```python
from build123d import *

# Parameters (mm, degrees)
SKETCH_W            = 80
SKETCH_H            = 120
PAD_DEPTH           = 3
SKETCH001_W         = 70
SKETCH001_H         = 110
POCKET_DEPTH        = 2
SKETCH002_W         = 62
SKETCH002_H         = 98.5
POCKET001_DEPTH     = 5
FILLET_R            = 2.54
CHAMFER_SIZE        = 1.99
SKETCH003_W         = 126
SKETCH003_H         = 60
PAD001_DEPTH        = 3
SKETCH004_W         = 80
SKETCH004_H         = 60
PAD002_DEPTH        = 3
CHAMFER001_SIZE     = 9.5
SKETCH005_R         = 1.8
POCKET002_DEPTH     = 8
FILLET001_R         = 2.99
SKETCH006_W         = 8
SKETCH006_H         = 10
PAD003_DEPTH        = 10
SKETCH007_W         = 8
SKETCH007_H         = 10
PAD004_DEPTH        = 20
SKETCH008_R         = 1.4
POCKET003_DEPTH     = 7
SKETCH009_R         = 1.4
POCKET004_DEPTH     = 7
CHAMFER002_SIZE     = 9.99
CHAMFER003_SIZE     = 9.99
CHAMFER004_SIZE     = 1.49
CHAMFER005_SIZE     = 6
CHAMFER005_FACE36_R = 1.4
POCKET005_DEPTH     = 2
POCKET005_FACE45_R  = 1.4
POCKET006_DEPTH     = 2
POCKET006_FACE2_R   = 1.4
POCKET007_DEPTH     = 2
POCKET007_FACE55_R  = 1.4
POCKET008_DEPTH     = 2
FILLET002_R         = 3.99


with BuildPart() as part:
    # Sketch → Pad (new body)
    with BuildSketch(Plane.XY):
        Rectangle(SKETCH_W, SKETCH_H)
    extrude(amount=PAD_DEPTH)

    # Sketch001 (on Face6 of Pad) → Pocket (cut)
    with BuildSketch(Plane.XY.offset(3)):
        Rectangle(SKETCH001_W, SKETCH001_H)
    extrude(amount=-POCKET_DEPTH, mode=Mode.SUBTRACT)

    # Sketch002 (on Face11 of Pocket) → Pocket001 (cut)
    with BuildSketch(Plane.XY.offset(1)):
        Rectangle(SKETCH002_W, SKETCH002_H)
    extrude(amount=-POCKET001_DEPTH, mode=Mode.SUBTRACT)

    # Fillet
    fillet_edges = [part.edges().sort_by_distance(p)[0] for p in [
        (-31, 49.25, 0.5),
        (31, 49.25, 0.5),
        (31, -49.25, 0.5),
        (-31, -49.25, 0.5),
    ]]
    fillet(fillet_edges, radius=FILLET_R)

    # Chamfer
    chamfer_edges = [part.edges().sort_by_distance(p)[0] for p in [
        (0, 55, 1),
        (35, 0, 1),
        (0, -55, 1),
        (-35, 0, 1),
    ]]
    chamfer(chamfer_edges, length=CHAMFER_SIZE)

    # Sketch003 (on Face22 of Chamfer) → Pad001 (join)
    with BuildSketch(Plane.YZ.offset(40)):
        with Locations((0, 30)):
            Rectangle(SKETCH003_W, SKETCH003_H)
    pad001 = extrude(amount=PAD001_DEPTH)

    # Mirrored: Pad001 across YZ
    add(pad001.mirror(Plane.YZ))

    # Sketch004 (on Face9 of Mirrored) → Pad002 (join)
    with BuildSketch(Plane(origin=(0, 60, 0), x_dir=(-1, 0, 0), z_dir=(0, 1, 0))):
        with Locations((0, 30)):
            Rectangle(SKETCH004_W, SKETCH004_H)
    pad002 = extrude(amount=PAD002_DEPTH)

    # Mirrored001: Pad002 across XZ
    add(pad002.mirror(Plane.XZ))

    # Chamfer001
    chamfer001_edges = [part.edges().sort_by_distance(p)[0] for p in [
        (-40, -60, 31.5),
        (-40, 60, 31.5),
        (40, 60, 31.5),
        (40, -60, 31.5),
    ]]
    chamfer(chamfer001_edges, length=CHAMFER001_SIZE)

    # Sketch005 (on Face4 of Chamfer001) → Pocket002 (cut)
    with BuildSketch(Plane.XY.offset(60)):
        with Locations((-38.403806, -58.403806)):
            Circle(SKETCH005_R)
        with Locations((38.403806, -58.403806)):
            Circle(SKETCH005_R)
    pocket002 = extrude(amount=-POCKET002_DEPTH, mode=Mode.SUBTRACT)

    # Mirrored002: Pocket002 across XZ
    add(pocket002.mirror(Plane.XZ), mode=Mode.SUBTRACT)

    # Fillet001
    fillet001_edges = [part.edges().sort_by_distance(p)[0] for p in [
        (-43, 63, 30),
        (-43, -63, 30),
        (43, -63, 30),
        (43, 63, 30),
    ]]
    fillet(fillet001_edges, radius=FILLET001_R)

    # Sketch006 (on Face21 of Fillet001) → Pad003 (join)
    with BuildSketch(Plane(origin=(0, -60, 0), x_dir=(-1, 0, 0), z_dir=(0, 1, 0))):
        with Locations((-25, 25)):
            Rectangle(SKETCH006_W, SKETCH006_H)
        with Locations((25, 25)):
            Rectangle(SKETCH006_W, SKETCH006_H)
    extrude(amount=PAD003_DEPTH)

    # Sketch007 (on Face10 of Pad003) → Pad004 (join)
    with BuildSketch(Plane.YZ.offset(-40)):
        with Locations((-4, 25)):
            Rectangle(SKETCH007_W, SKETCH007_H)
    pad004 = extrude(amount=PAD004_DEPTH)

    # Sketch008 (on Face41 of Pad004) → Pocket003 (cut)
    with BuildSketch(Plane.XY.offset(30)):
        with Locations((-25, -54)):
            Circle(SKETCH008_R)
    pocket003 = extrude(amount=-POCKET003_DEPTH, mode=Mode.SUBTRACT)

    # Mirrored003: Pocket003 across Sketch008 V_Axis
    add(pocket003.mirror(Plane(origin=(0, 0, 30), x_dir=(0, 0, 1), z_dir=(1, 0, 0))), mode=Mode.SUBTRACT)

    # Sketch009 (on Face26 of Mirrored003) → Pocket004 (cut)
    with BuildSketch(Plane.XY.offset(30)):
        with Locations((-25, -4)):
            Circle(SKETCH009_R)
    pocket004 = extrude(amount=-POCKET004_DEPTH, mode=Mode.SUBTRACT)

    # Mirrored004: Pad004 across YZ
    add(pad004.mirror(Plane.YZ))

    # Mirrored005: Pocket004 across Sketch009 V_Axis
    add(pocket004.mirror(Plane(origin=(0, 0, 30), x_dir=(0, 0, 1), z_dir=(1, 0, 0))), mode=Mode.SUBTRACT)

    # Chamfer002
    chamfer002_edges = [part.edges().sort_by_distance(p)[0] for p in [
        (25, -60, 20),
        (-25, -60, 20),
    ]]
    chamfer(chamfer002_edges, length=CHAMFER002_SIZE)

    # Chamfer003
    chamfer003_edges = [part.edges().sort_by_distance(p)[0] for p in [
        (40, -4, 20),
        (-40, -4, 20),
    ]]
    chamfer(chamfer003_edges, length=CHAMFER003_SIZE)

    # Chamfer004
    chamfer004_edges = [part.edges().sort_by_distance(p)[0] for p in [
        (29, -60, 15.005),
        (29, -60, 25),
        (-29, -60, 15.005),
        (-21, -60, 15.005),
        (21, -60, 15.005),
    ]]
    chamfer(chamfer004_edges, length=CHAMFER004_SIZE)

    # Chamfer005
    chamfer005_edges = [part.edges().sort_by_distance(p)[0] for p in [
        (-40, 0, 15.005),
        (-40, -8, 15.005),
        (40, -8, 15.005),
        (40, 0, 15.005),
    ]]
    chamfer(chamfer005_edges, length=CHAMFER005_SIZE)

    # Chamfer005 Face36 → Pocket005 (cut)
    with BuildSketch(Plane(origin=(31.679222, -4, 30), x_dir=(0, 1, 0), z_dir=(0, 0, 1))):
        Polygon((-4, 11.679222), (-4, -2.320778), (-10, -8.320778), (-4, -8.320778), (4, -8.320778), (10, -8.320778), (4, -2.320778), (4, 11.679222), align=None)
        with Locations((0, 6.679222)):
            Circle(CHAMFER005_FACE36_R, mode=Mode.SUBTRACT)
    extrude(amount=-POCKET005_DEPTH, mode=Mode.SUBTRACT)

    # Pocket005 Face45 → Pocket006 (cut)
    with BuildSketch(Plane(origin=(25, -55.212396, 30), x_dir=(0, 1, 0), z_dir=(0, 0, 1))):
        Polygon((-3.297604, -4), (5.212396, -4), (5.212396, 4), (-3.297604, 4), (-4.787604, 5.49), (-4.787604, 4), (-4.787604, -4), (-4.787604, -5.49), align=None)
        with Locations((1.212396, 0)):
            Circle(POCKET005_FACE45_R, mode=Mode.SUBTRACT)
    extrude(amount=-POCKET006_DEPTH, mode=Mode.SUBTRACT)

    # Pocket006 Face2 → Pocket007 (cut)
    with BuildSketch(Plane(origin=(-31.679222, -4, 30), x_dir=(0, 1, 0), z_dir=(0, 0, 1))):
        Polygon((-4, 2.320778), (-4, -11.679222), (4, -11.679222), (4, 2.320778), (10, 8.320778), (4, 8.320778), (-4, 8.320778), (-10, 8.320778), align=None)
        with Locations((0, -6.679222)):
            Circle(POCKET006_FACE2_R, mode=Mode.SUBTRACT)
    extrude(amount=-POCKET007_DEPTH, mode=Mode.SUBTRACT)

    # Pocket007 Face55 → Pocket008 (cut)
    with BuildSketch(Plane(origin=(-25, -55.212396, 30), x_dir=(0, 1, 0), z_dir=(0, 0, 1))):
        Polygon((-3.297604, -4), (5.212396, -4), (5.212396, 4), (-3.297604, 4), (-4.787604, 5.49), (-4.787604, 4), (-4.787604, -4), (-4.787604, -5.49), align=None)
        with Locations((1.212396, 0)):
            Circle(POCKET007_FACE55_R, mode=Mode.SUBTRACT)
    extrude(amount=-POCKET008_DEPTH, mode=Mode.SUBTRACT)

    # Fillet002
    fillet002_edges = [part.edges().sort_by_distance(p)[0] for p in [
        (20, 0, 24),
        (20, -8, 24),
        (-20, -8, 24),
        (-20, 0, 24),
        (-29, -50, 24),
        (-21, -50, 24),
        (21, -50, 24),
        (29, -50, 24),
    ]]
    fillet(fillet002_edges, radius=FILLET002_R)


solid = part.part
```
Geometry check sheet. Reference: the model listing, model coordinates, mm. A direction names the side the tool comes from. Give positions to 0.01 mm unless a question says otherwise; leave off trailing zeros. Loops run counter-clockwise (first coordinate to the right, second up) from the corner with the lowest first, then second, coordinate; pieces in that order, holes last. Notation, with made-up numbers: M -2.75,77.25 L 3.25,77.25 A25 ccw 3.25,107.25 Z; hole C -15.75,74 d8. An arc over 180 degrees is marked long. Write item = value, one per line. Start each with the question number.
1. Tool access check on faces 1 (the face through (-25, -54, 23)), 2 (the face through (-43, -1, 30)), 3 (the face through (25.08, -54.94, 15.07)), 4 (the face through (-21.14, -6.8, 24.06)). Record the directions out of +Z, -Z, +X, -X, +Y, -Y that give a thin tool (end or side, any length) a straight path to the whole face; none if there is none.
2. Draft check along X on faces 5 (the face through (37, 3, 21)), 6 (the face through (-42.15, 62.1, 30.42)), 7 (the face through (39, 1, 0)). Enter one of: +X half, -X half, draft (parallel to the pull), parting line (faces both ways), or undercut.
3. Section check C-C, the plane z = 8. Enter the section's corners in (x, y), plus the area to 3 significant figures.
4. Go/stop test with flat-tipped pins: P1, Ø2, axis at x = 25, y = -54.5, coming from the +Z side; P2, Ø0.8, axis at x = -24.5, y = -3.5, coming from the +Z side. Record where each tip stops, or that it passes through.
5. Section check D-D, the plane z = 55.5. Enter the section's corners in (x, y), plus the area to 3 significant figures.
6. Thickness scan on probe 1 along Y at (x, z) = (25, 24.7); probe 2 along X at (y, z) = (-4, 26.6); probe 3 along X at (y, z) = (-5, 57). Record the ranges inside material, lowest first.
Values follow:
q1.face_1 = +Z
q1.face_2 = +Z, -Z, -X, +Y, -Y
q1.face_3 = none
q1.face_4 = +Z, -Z
q2.face_5 = undercut
q2.face_6 = -X half
q2.face_7 = draft
q3.outline = M -43,-60.01 A2.99 ccw -40.01,-63 L 40.01,-63 A2.99 ccw 43,-60.01 L 43,60.01 A2.99 ccw 40.01,63 L -40.01,63 A2.99 ccw -43,60.01 Z; hole M -40,-50.5 L -30.5,-60 L 30.5,-60 L 40,-50.5 L 40,50.5 L 30.5,60 L -30.5,60 L -40,50.5 Z
q3.area = 1,410 mm^2
q4.P1 = 28
q4.P2 = 23
q5.outline = M -43,-60.01 A2.99 ccw -40.01,-63 L 40.01,-63 A2.99 ccw 43,-60.01 L 43,60.01 A2.99 ccw 40.01,63 L -40.01,63 A2.99 ccw -43,60.01 Z; hole C -38.4,-58.4 d3.6; hole C -38.4,58.4 d3.6; hole M -40,-50.5 L -30.5,-60 L 30.5,-60 L 40,-50.5 L 40,50.5 L 30.5,60 L -30.5,60 L -40,50.5 Z; hole C 38.4,-58.4 d3.6; hole C 38.4,58.4 d3.6
q5.area = 1,370 mm^2
q6.probe_1 = -63 to -55.4, -52.6 to -50, -8 to -5.4, -2.6 to 0, 60 to 63
q6.probe_2 = -43 to -26.4, -23.6 to -20, 20 to 23.6, 26.4 to 43
q6.probe_3 = -43 to -40, 40 to 43
